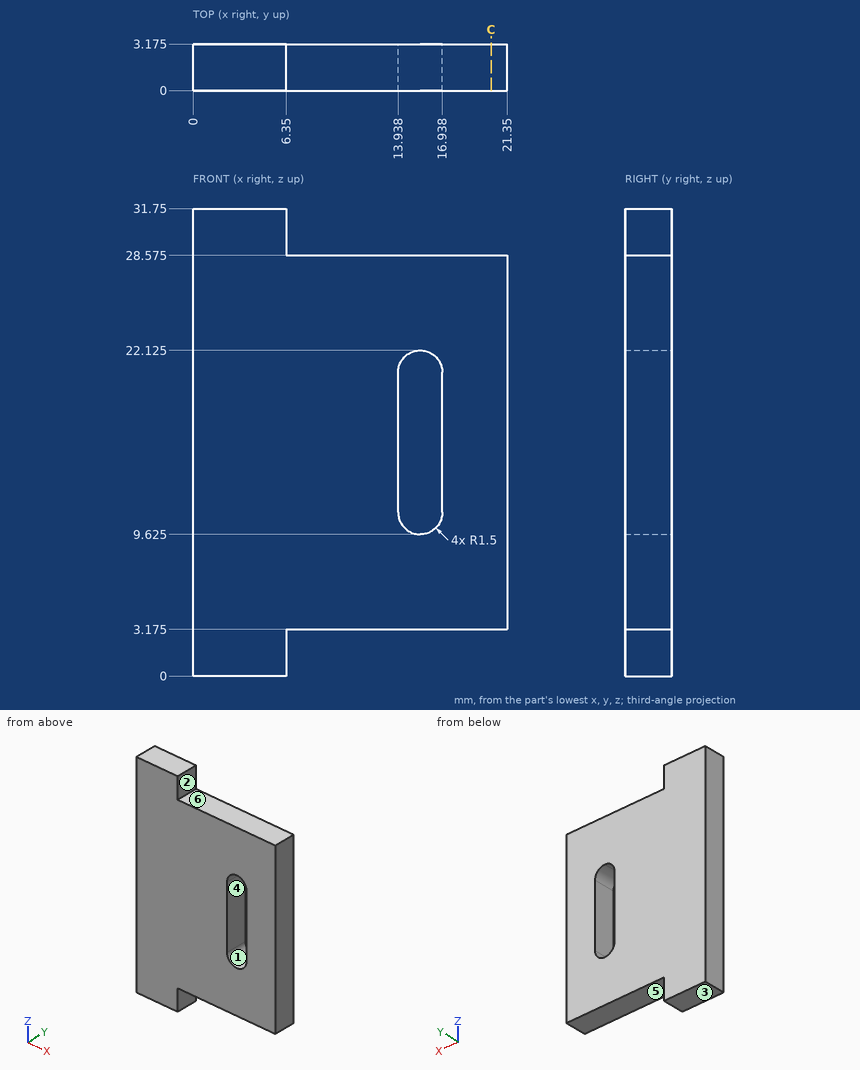
Here's the drawing with two shaded views (mm, measured from the low corner). I have some questions. A direction names the side the tool comes from. Coordinates: 2 decimals unless noted, no trailing zeros. Write each loop counter-clockwise with the first axis right and the second up, starting at its lowest first coordinate (ties: lowest second). Pieces come first, ordered by that corner, then holes. Notation, with made-up numbers: (-14, 33) -> (6, 33) arc R33 cw to (6, 66) -> close; hole circle Ø3 at (-20.5, -27). An arc over 180 degrees is marked (long way). Write item = value, one per line. Start each with the question number.
(1) Which directions (+Z, -Z, +X, -X, +Y, -Y) give clear straight access to the entire face, cutting with the end or side of a thin tool? Please do the marked faces 4, 5 and 6.
(2) I need wall thicknesses on line 1 (X direction, y = 1.6, z = 18); line 2 (Z direction, x = 8.75, y = 3) (1 decimal); line 3 (X direction, y = 0.6, z = 30). Which ranges of each line are inside material? Lowest first, please. Write a range as [from, to].
(3) I want a section at C-C (x = 20.25). Please give me the cut outline in (y, z) (1 decimal).
(4) We'd pull the mould along Z, two halves only. Please class the marked faces 1, 2 and 3: released by +Z, released by -Z, zero draft, split by the parting line, or undercut.
(5) Will this pin go through, and if not, where does the flat tip stop? pin 1 (4 mm diameter, centred on x = 9, z = 12.5, fed in from -Y).
Result set:
q1.face_4 = +Y, -Y
q1.face_5 = -Z, +X, +Y, -Y
q1.face_6 = +Z, +X, +Y, -Y
q2.line_1 = [0, 13.94], [16.94, 21.35]
q2.line_2 = [3.2, 28.6]
q2.line_3 = [0, 6.35]
q3.outline = (0, 3.2) -> (3.2, 3.2) -> (3.2, 28.6) -> (0, 28.6) -> close
q4.face_1 = undercut
q4.face_2 = zero draft
q4.face_3 = released by -Z
q5.pin_1 = 0
